from build123d import *

# Parameters (mm, degrees)
BOSS_EXTRUDE1_DEPTH = 139.7
SKETCH2_R           = 2.0828
CUT_EXTRUDE1_DEPTH  = 164.110921143
CUT_EXTRUDE3_REACH  = 151.165
SKETCH4_R           = 2.0193
SKETCH5_R           = 9.525
CUT_EXTRUDE4_DEPTH  = 149.188049505


with BuildPart() as part:
    # Sketch1 → Boss-Extrude1 (new, symmetric)
    with BuildSketch(Plane(origin=(0, 0, 0), x_dir=(0, 0, -1), z_dir=(1, 0, 0))):
        Polygon((0, 38.1), (0, -38.1), (35.814, -38.1), (35.814, -33.782), (4.318, -33.782), (4.318, 33.782), (35.814, 33.782), (35.814, 38.1), align=None)
    extrude(amount=BOSS_EXTRUDE1_DEPTH, both=True)

    # Sketch2 → Cut-Extrude1 (cut, through all)
    with BuildSketch(Plane(origin=(0, 38.1, 0), x_dir=(1, 0, 0), z_dir=(0, 1, 0))):
        with Locations(Location((-133.35, 27.94, 0), (0, 0, 270))):
            Circle(SKETCH2_R)
        with Locations(Location((-133.35, 15.24, 0), (0, 0, 270))):
            Circle(SKETCH2_R)
        with Locations(Location((-120.65, 27.94, 0), (0, 0, 270))):
            Circle(SKETCH2_R)
        with Locations(Location((-120.65, 15.24, 0), (0, 0, 270))):
            Circle(SKETCH2_R)
        with Locations(Location((-107.95, 27.94, 0), (0, 0, 270))):
            Circle(SKETCH2_R)
        with Locations(Location((-107.95, 15.24, 0), (0, 0, 270))):
            Circle(SKETCH2_R)
        with Locations(Location((-95.25, 27.94, 0), (0, 0, 270))):
            Circle(SKETCH2_R)
        with Locations(Location((-95.25, 15.24, 0), (0, 0, 270))):
            Circle(SKETCH2_R)
        with Locations(Location((-82.55, 27.94, 0), (0, 0, 270))):
            Circle(SKETCH2_R)
        with Locations(Location((-82.55, 15.24, 0), (0, 0, 270))):
            Circle(SKETCH2_R)
        with Locations(Location((-69.85, 27.94, 0), (0, 0, 270))):
            Circle(SKETCH2_R)
        with Locations(Location((-69.85, 15.24, 0), (0, 0, 270))):
            Circle(SKETCH2_R)
        with Locations(Location((-57.15, 27.94, 0), (0, 0, 270))):
            Circle(SKETCH2_R)
        with Locations(Location((-57.15, 15.24, 0), (0, 0, 270))):
            Circle(SKETCH2_R)
        with Locations(Location((-44.45, 27.94, 0), (0, 0, 270))):
            Circle(SKETCH2_R)
        with Locations(Location((-44.45, 15.24, 0), (0, 0, 270))):
            Circle(SKETCH2_R)
        with Locations(Location((-31.75, 27.94, 0), (0, 0, 270))):
            Circle(SKETCH2_R)
        with Locations(Location((-31.75, 15.24, 0), (0, 0, 270))):
            Circle(SKETCH2_R)
        with Locations(Location((-19.05, 27.94, 0), (0, 0, 270))):
            Circle(SKETCH2_R)
        with Locations(Location((-19.05, 15.24, 0), (0, 0, 270))):
            Circle(SKETCH2_R)
        with Locations(Location((-6.35, 27.94, 0), (0, 0, 270))):
            Circle(SKETCH2_R)
        with Locations(Location((-6.35, 15.24, 0), (0, 0, 270))):
            Circle(SKETCH2_R)
        with Locations(Location((6.35, 27.94, 0), (0, 0, 270))):
            Circle(SKETCH2_R)
        with Locations(Location((6.35, 15.24, 0), (0, 0, 270))):
            Circle(SKETCH2_R)
        with Locations(Location((19.05, 27.94, 0), (0, 0, 270))):
            Circle(SKETCH2_R)
        with Locations(Location((19.05, 15.24, 0), (0, 0, 270))):
            Circle(SKETCH2_R)
        with Locations(Location((31.75, 27.94, 0), (0, 0, 270))):
            Circle(SKETCH2_R)
        with Locations(Location((31.75, 15.24, 0), (0, 0, 270))):
            Circle(SKETCH2_R)
        with Locations(Location((44.45, 27.94, 0), (0, 0, 270))):
            Circle(SKETCH2_R)
        with Locations(Location((44.45, 15.24, 0), (0, 0, 270))):
            Circle(SKETCH2_R)
        with Locations(Location((57.15, 27.94, 0), (0, 0, 270))):
            Circle(SKETCH2_R)
        with Locations(Location((57.15, 15.24, 0), (0, 0, 270))):
            Circle(SKETCH2_R)
        with Locations(Location((69.85, 27.94, 0), (0, 0, 270))):
            Circle(SKETCH2_R)
        with Locations(Location((69.85, 15.24, 0), (0, 0, 270))):
            Circle(SKETCH2_R)
        with Locations(Location((82.55, 27.94, 0), (0, 0, 270))):
            Circle(SKETCH2_R)
        with Locations(Location((82.55, 15.24, 0), (0, 0, 270))):
            Circle(SKETCH2_R)
        with Locations(Location((95.25, 27.94, 0), (0, 0, 270))):
            Circle(SKETCH2_R)
        with Locations(Location((95.25, 15.24, 0), (0, 0, 270))):
            Circle(SKETCH2_R)
        with Locations(Location((107.95, 27.94, 0), (0, 0, 270))):
            Circle(SKETCH2_R)
        with Locations(Location((107.95, 15.24, 0), (0, 0, 270))):
            Circle(SKETCH2_R)
        with Locations(Location((120.65, 27.94, 0), (0, 0, 270))):
            Circle(SKETCH2_R)
        with Locations(Location((120.65, 15.24, 0), (0, 0, 270))):
            Circle(SKETCH2_R)
        with Locations(Location((133.35, 27.94, 0), (0, 0, 270))):
            Circle(SKETCH2_R)
        with Locations(Location((133.35, 15.24, 0), (0, 0, 270))):
            Circle(SKETCH2_R)
    extrude(amount=-CUT_EXTRUDE1_DEPTH, mode=Mode.SUBTRACT)

    # Sketch4 → Cut-Extrude3 (cut, up to next)
    with BuildSketch(Plane.XY, mode=Mode.PRIVATE) as cut_extrude3_sk1:
        with Locations((-71.016697469, 3.925)):
            Circle(SKETCH4_R)
    cut_extrude3_tool1 = extrude(cut_extrude3_sk1.sketch, amount=-CUT_EXTRUDE3_REACH, mode=Mode.PRIVATE) & part.part
    # Sketch4 → Cut-Extrude3 (cut, up to next)
    with BuildSketch(Plane.XY, mode=Mode.PRIVATE) as cut_extrude3_sk2:
        with Locations((-45.616697469, -27.825)):
            Circle(SKETCH4_R)
    cut_extrude3_tool2 = extrude(cut_extrude3_sk2.sketch, amount=-CUT_EXTRUDE3_REACH, mode=Mode.PRIVATE) & part.part
    # Sketch4 → Cut-Extrude3 (cut, up to next)
    with BuildSketch(Plane.XY, mode=Mode.PRIVATE) as cut_extrude3_sk3:
        with Locations((-45.616697469, 3.925)):
            Circle(SKETCH4_R)
    cut_extrude3_tool3 = extrude(cut_extrude3_sk3.sketch, amount=-CUT_EXTRUDE3_REACH, mode=Mode.PRIVATE) & part.part
    # Sketch4 → Cut-Extrude3 (cut, up to next)
    with BuildSketch(Plane.XY, mode=Mode.PRIVATE) as cut_extrude3_sk4:
        with Locations((-71.016697469, -27.825)):
            Circle(SKETCH4_R)
    cut_extrude3_tool4 = extrude(cut_extrude3_sk4.sketch, amount=-CUT_EXTRUDE3_REACH, mode=Mode.PRIVATE) & part.part
    # Sketch4 → Cut-Extrude3 (cut, up to next)
    with BuildSketch(Plane.XY, mode=Mode.PRIVATE) as cut_extrude3_sk5:
        with Locations((45.616697469, -27.825)):
            Circle(SKETCH4_R)
    cut_extrude3_tool5 = extrude(cut_extrude3_sk5.sketch, amount=-CUT_EXTRUDE3_REACH, mode=Mode.PRIVATE) & part.part
    # Sketch4 → Cut-Extrude3 (cut, up to next)
    with BuildSketch(Plane.XY, mode=Mode.PRIVATE) as cut_extrude3_sk6:
        with Locations((71.016697469, -27.825)):
            Circle(SKETCH4_R)
    cut_extrude3_tool6 = extrude(cut_extrude3_sk6.sketch, amount=-CUT_EXTRUDE3_REACH, mode=Mode.PRIVATE) & part.part
    # Sketch4 → Cut-Extrude3 (cut, up to next)
    with BuildSketch(Plane.XY, mode=Mode.PRIVATE) as cut_extrude3_sk7:
        with Locations((71.016697469, 3.925)):
            Circle(SKETCH4_R)
    cut_extrude3_tool7 = extrude(cut_extrude3_sk7.sketch, amount=-CUT_EXTRUDE3_REACH, mode=Mode.PRIVATE) & part.part
    # Sketch4 → Cut-Extrude3 (cut, up to next)
    with BuildSketch(Plane.XY, mode=Mode.PRIVATE) as cut_extrude3_sk8:
        with Locations((45.616697469, 3.925)):
            Circle(SKETCH4_R)
    cut_extrude3_tool8 = extrude(cut_extrude3_sk8.sketch, amount=-CUT_EXTRUDE3_REACH, mode=Mode.PRIVATE) & part.part
    add(cut_extrude3_tool1.solids().sort_by_distance((-71.016697, 3.925, 0))[0], mode=Mode.SUBTRACT)
    add(cut_extrude3_tool2.solids().sort_by_distance((-45.616697, -27.825, 0))[0], mode=Mode.SUBTRACT)
    add(cut_extrude3_tool3.solids().sort_by_distance((-45.616697, 3.925, 0))[0], mode=Mode.SUBTRACT)
    add(cut_extrude3_tool4.solids().sort_by_distance((-71.016697, -27.825, 0))[0], mode=Mode.SUBTRACT)
    add(cut_extrude3_tool5.solids().sort_by_distance((45.616697, -27.825, 0))[0], mode=Mode.SUBTRACT)
    add(cut_extrude3_tool6.solids().sort_by_distance((71.016697, -27.825, 0))[0], mode=Mode.SUBTRACT)
    add(cut_extrude3_tool7.solids().sort_by_distance((71.016697, 3.925, 0))[0], mode=Mode.SUBTRACT)
    add(cut_extrude3_tool8.solids().sort_by_distance((45.616697, 3.925, 0))[0], mode=Mode.SUBTRACT)

    # Sketch5 → Cut-Extrude4 (cut, through all)
    with BuildSketch(Plane(origin=(0, 0, -4.318), x_dir=(-1, 0, 0), z_dir=(0, 0, -1))):
        with Locations((104.14, 0)):
            Circle(SKETCH5_R)
        with Locations((-104.14, 0)):
            Circle(SKETCH5_R)
    extrude(amount=-CUT_EXTRUDE4_DEPTH, mode=Mode.SUBTRACT)


solid = part.part
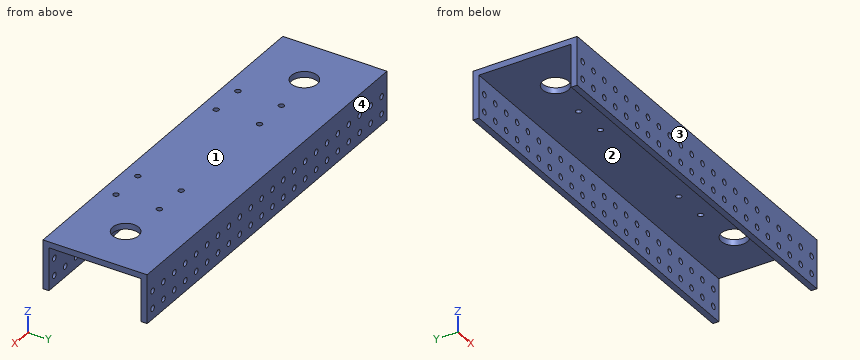
The listing builds one solid part. Answer for the finished solid, in the listing's coordinates (mm). Face numbers are marked on the shaded views. Coordinates: 2 decimals unless noted, no trailing zeros. Order: outer loops, then holes, each group sorted by start corner. A loop starts at its lowest first (then second) coordinate and runs counter-clockwise, first axis right, second up.
Q1. Given P1, Ø4.5, axis at x = 71.02, y = -27.82, coming from the -Z side; P2, Ø3.5, axis at x = 31.75, z = -15.24, coming from the +Y side, each flat-ended and moving along its own axis, determine where each tip first touches the part or whether it passes through.
Q2. Consider line 1 (Z direction, x = -19, y = 37); line 2 (Y direction, x = -22, z = -13); line 3 (Z direction, x = -82, y = 36). Determine where each line is inside the solid, lowest interval first.
Q3. A cutting plane is placed at B-B, the plane x = 100. Write down the section's boundary in (y, z), and give its area (3 significant figures).
Q4. A cutting plane is placed at C-C, the plane y = 28.5. Write down the section's boundary in (x, z), and give its area (3 significant figures).
Q5. A cutting plane is placed at A-A, the plane x = -77. Write down the section's boundary in (y, z).
Q6. For a pull along Y with two mould halves and no side action, classify the marked faces 1, 2, 3 and 4 as pulls with the +Y half, pulls with the -Y half, needs draft (parallel to the pull), parting line crosses it, or undercut.
Answers follow:
1. P1: stops at z = -4.32
1. P2: passes through
2. line 1: z = -35.81 to -30.02, -25.86 to -17.32, -13.16 to 0
2. line 2: y = -38.1 to -33.78, 33.78 to 38.1
2. line 3: z = -35.81 to -29.95, -25.93 to -17.25, -13.23 to 0
3. outline: (-38.1, -35.81) - (-33.78, -35.81) - (-33.78, -4.32) - (-8.58, -4.32) - (-8.58, 0) - (-38.1, 0) - close; (8.58, -4.32) - (33.78, -4.32) - (33.78, -35.81) - (38.1, -35.81) - (38.1, 0) - (8.58, 0) - close
3. area: 527 mm2
4. outline: (-139.7, -4.32) - (139.7, -4.32) - (139.7, 0) - (-139.7, 0) - close
4. area: 1,210 mm2
5. outline: (-38.1, -35.81) - (-33.78, -35.81) - (-33.78, -4.32) - (33.78, -4.32) - (33.78, -35.81) - (38.1, -35.81) - (38.1, 0) - (-38.1, 0) - close
6. face 1: needs draft
6. face 2: undercut
6. face 3: pulls with the -Y half
6. face 4: pulls with the +Y half
